from build123d import *

# Parameters (mm, degrees)
SKETCH_W        = 106.6
SKETCH_H        = 40
PAD_DEPTH       = 180
SKETCH001_W     = 102.8
SKETCH001_H     = 176.2
POCKET_DEPTH    = 38.1
SKETCH002_W     = 102.8
SKETCH002_H     = 1.9
POCKET001_DEPTH = 38.1
SKETCH003_W     = 50
SKETCH003_H     = 15
POCKET002_DEPTH = 5
SKETCH004_W     = 22
SKETCH004_H     = 20
POCKET003_DEPTH = 5
SKETCH005_W     = 75
SKETCH005_H     = 22
POCKET004_DEPTH = 5
SKETCH006_R     = 4
SKETCH006_R_2   = 4.25
POCKET005_DEPTH = 5
CHAMFER_SIZE    = 5
CHAMFER001_SIZE = 5
SKETCH007_W     = 5
SKETCH007_H     = 10
POCKET006_DEPTH = 5
SKETCH008_W     = 5
SKETCH008_H     = 10
POCKET007_DEPTH = 5
SKETCH009_W     = 19.8
SKETCH009_H     = 10
POCKET008_DEPTH = 5
SKETCH010_W     = 40
SKETCH010_H     = 5
PAD001_DEPTH    = 5
CHAMFER002_SIZE = 3.099
CHAMFER003_SIZE = 3
SKETCH011_W     = 40
SKETCH011_H     = 5
PAD002_DEPTH    = 5
CHAMFER004_SIZE = 3.099
CHAMFER005_SIZE = 3
SKETCH012_W     = 3.5
SKETCH012_H     = 22
POCKET009_DEPTH = 5
SKETCH013_W     = 3.5
SKETCH013_H     = 22
POCKET010_DEPTH = 5
SKETCH014_W     = 29
SKETCH014_H     = 50
POCKET011_DEPTH = 5
SKETCH015_W     = 102.8
SKETCH015_H     = 12
POCKET012_DEPTH = 5
SKETCH016_W     = 10
SKETCH016_H     = 12.5
POCKET013_DEPTH = 5
SKETCH017_W     = 40
SKETCH017_H     = 4
PAD003_DEPTH    = 4
CHAMFER006_SIZE = 3.099
CHAMFER007_SIZE = 1.99
SKETCH018_R     = 2.5
POCKET014_DEPTH = 5
SKETCH019_W     = 10
SKETCH019_H     = 8
POCKET015_DEPTH = 5


with BuildPart() as part:
    # Sketch → Pad (new body)
    with BuildSketch(Plane.XY):
        Rectangle(SKETCH_W, SKETCH_H)
    extrude(amount=PAD_DEPTH)

    # Sketch001 (on Face1 of Pad) → Pocket (cut)
    with BuildSketch(Plane(origin=(0, 20, 0), x_dir=(-1, 0, 0), z_dir=(0, 1, 0))):
        with Locations((0, 90)):
            Rectangle(SKETCH001_W, SKETCH001_H)
    extrude(amount=-POCKET_DEPTH, mode=Mode.SUBTRACT)

    # Sketch002 (on Face1 of Pocket) → Pocket001 (cut)
    with BuildSketch(Plane(origin=(0, 20, 0), x_dir=(-1, 0, 0), z_dir=(0, 1, 0))):
        with Locations((0, 0.95)):
            Rectangle(SKETCH002_W, SKETCH002_H)
    extrude(amount=-POCKET001_DEPTH, mode=Mode.SUBTRACT)

    # Sketch003 (on Face11 of Pocket001) → Pocket002 (cut)
    with BuildSketch(Plane.XZ.offset(20)):
        with Locations((0, 7.5)):
            Rectangle(SKETCH003_W, SKETCH003_H)
    extrude(amount=-POCKET002_DEPTH, mode=Mode.SUBTRACT)

    # Sketch004 (on Face9 of Pocket002) → Pocket003 (cut)
    with BuildSketch(Plane.YZ.offset(53.3)):
        with Locations((0, 57.78728)):
            Rectangle(SKETCH004_W, SKETCH004_H)
    extrude(amount=-POCKET003_DEPTH, mode=Mode.SUBTRACT)

    # Sketch005 (on Face10 of Pocket003) → Pocket004 (cut)
    with BuildSketch(Plane.XY.offset(180)):
        Rectangle(SKETCH005_W, SKETCH005_H)
    extrude(amount=-POCKET004_DEPTH, mode=Mode.SUBTRACT)

    # Sketch006 (on Face12 of Pocket004) → Pocket005 (cut)
    with BuildSketch(Plane.XZ.offset(20)):
        with Locations((39.85, 19.5)):
            Circle(SKETCH006_R)
        with Locations((39.85, 38.2)):
            Circle(SKETCH006_R_2)
    extrude(amount=-POCKET005_DEPTH, mode=Mode.SUBTRACT)

    # Chamfer
    chamfer_edges = [part.edges().sort_by_distance(p)[0] for p in [
        (-51.4, -18.1, 90),
        (-51.4, 0.95, 178.1),
        (0, -18.1, 178.1),
        (51.4, -18.1, 90),
        (51.4, 0.95, 178.1),
    ]]
    chamfer(chamfer_edges, length=CHAMFER_SIZE)

    # Chamfer001
    chamfer001_edges = [part.edges().sort_by_distance(p)[0] for p in [
        (53.3, -20, 90),
        (-53.3, -20, 90),
        (0, -20, 180),
        (53.3, 0, 180),
        (-53.3, 0, 180),
    ]]
    chamfer(chamfer001_edges, length=CHAMFER001_SIZE)

    # Sketch007 (on Face9 of Chamfer001) → Pocket006 (cut)
    with BuildSketch(Plane.YZ.offset(53.3)):
        with Locations((7.5, 145)):
            Rectangle(SKETCH007_W, SKETCH007_H)
        with Locations((7.5, 35)):
            Rectangle(SKETCH007_W, SKETCH007_H)
    extrude(amount=-POCKET006_DEPTH, mode=Mode.SUBTRACT)

    # Sketch008 (on Face2 of Pocket006) → Pocket007 (cut)
    with BuildSketch(Plane(origin=(-53.3, 0, 0), x_dir=(0, -1, 0), z_dir=(-1, 0, 0))):
        with Locations((-7.5, 145)):
            Rectangle(SKETCH008_W, SKETCH008_H)
        with Locations((-7.5, 35)):
            Rectangle(SKETCH008_W, SKETCH008_H)
    extrude(amount=-POCKET007_DEPTH, mode=Mode.SUBTRACT)

    # Sketch009 (on Face2 of Pocket007) → Pocket008 (cut)
    with BuildSketch(Plane(origin=(-53.3, 0, 0), x_dir=(0, -1, 0), z_dir=(-1, 0, 0))):
        with Locations((-10.1, 17.5)):
            Rectangle(SKETCH009_W, SKETCH009_H)
    extrude(amount=-POCKET008_DEPTH, mode=Mode.SUBTRACT)

    # Sketch010 (on Face4 of Pocket008) → Pad001 (join)
    with BuildSketch(Plane.YZ.offset(-51.4)):
        with Locations((0, 2.5)):
            Rectangle(SKETCH010_W, SKETCH010_H)
    extrude(amount=PAD001_DEPTH)

    # Chamfer002
    chamfer002_edges = [part.edges().sort_by_distance(p)[0] for p in [
        (-51.4, -20, 2.5),
    ]]
    chamfer(chamfer002_edges, length=CHAMFER002_SIZE)

    # Chamfer003
    chamfer003_edges = [part.edges().sort_by_distance(p)[0] for p in [
        (-46.4, 0.95, 5),
    ]]
    chamfer(chamfer003_edges, length=CHAMFER003_SIZE)

    # Sketch011 (on Face27 of Chamfer003) → Pad002 (join)
    with BuildSketch(Plane(origin=(51.4, 0, 0), x_dir=(0, -1, 0), z_dir=(-1, 0, 0))):
        with Locations((0, 2.5)):
            Rectangle(SKETCH011_W, SKETCH011_H)
    extrude(amount=PAD002_DEPTH)

    # Chamfer004
    chamfer004_edges = [part.edges().sort_by_distance(p)[0] for p in [
        (51.4, -20, 2.5),
    ]]
    chamfer(chamfer004_edges, length=CHAMFER004_SIZE)

    # Chamfer005
    chamfer005_edges = [part.edges().sort_by_distance(p)[0] for p in [
        (46.4, 0.95, 5),
    ]]
    chamfer(chamfer005_edges, length=CHAMFER005_SIZE)

    # Sketch012 (on Face15 of Chamfer005) → Pocket009 (cut)
    with BuildSketch(Plane.YZ.offset(53.3)):
        with Locations((18.25, 102)):
            Rectangle(SKETCH012_W, SKETCH012_H)
    extrude(amount=-POCKET009_DEPTH, mode=Mode.SUBTRACT)

    # Sketch013 (on Face52 of Pocket009) → Pocket010 (cut)
    with BuildSketch(Plane(origin=(-53.3, 0, 0), x_dir=(0, -1, 0), z_dir=(-1, 0, 0))):
        with Locations((-18.25, 102)):
            Rectangle(SKETCH013_W, SKETCH013_H)
    extrude(amount=-POCKET010_DEPTH, mode=Mode.SUBTRACT)

    # Sketch014 (on Face52 of Pocket010) → Pocket011 (cut)
    with BuildSketch(Plane(origin=(-53.3, 0, 0), x_dir=(0, -1, 0), z_dir=(-1, 0, 0))):
        with Locations((-5.5, 101)):
            Rectangle(SKETCH014_W, SKETCH014_H)
    extrude(amount=-POCKET011_DEPTH, mode=Mode.SUBTRACT)

    # Sketch015 (on Face6 of Pocket011) → Pocket012 (cut)
    with BuildSketch(Plane(origin=(0, 0, 0), x_dir=(1, 0, 0), z_dir=(0, 0, -1))):
        with Locations((0, -14)):
            Rectangle(SKETCH015_W, SKETCH015_H)
    extrude(amount=-POCKET012_DEPTH, mode=Mode.SUBTRACT)

    # Sketch016 (on Face37 of Pocket012) → Pocket013 (cut)
    with BuildSketch(Plane(origin=(-53.3, 0, 0), x_dir=(0, -1, 0), z_dir=(-1, 0, 0))):
        with Locations((-15, 6.25)):
            Rectangle(SKETCH016_W, SKETCH016_H)
    extrude(amount=-POCKET013_DEPTH, mode=Mode.SUBTRACT)

    # Sketch017 (on Face32 of Pocket013) → Pad003 (join)
    with BuildSketch(Plane.YZ.offset(-51.4)):
        with Locations((0, 71)):
            Rectangle(SKETCH017_W, SKETCH017_H)
        with Locations((0, 131)):
            Rectangle(SKETCH017_W, SKETCH017_H)
    extrude(amount=PAD003_DEPTH)

    # Chamfer006
    chamfer006_edges = [part.edges().sort_by_distance(p)[0] for p in [
        (-51.4, -20, 131),
        (-51.4, -20, 71),
    ]]
    chamfer(chamfer006_edges, length=CHAMFER006_SIZE)

    # Chamfer007
    chamfer007_edges = [part.edges().sort_by_distance(p)[0] for p in [
        (-47.4, 1.45, 129),
        (-47.4, 1.45, 133),
        (-47.4, 1.45, 73),
        (-47.4, 1.45, 69),
    ]]
    chamfer(chamfer007_edges, length=CHAMFER007_SIZE)

    # Sketch018 (on Face66 of Chamfer007) → Pocket014 (cut)
    with BuildSketch(Plane.XZ.offset(20)):
        with Locations((8.85, 19.5)):
            Circle(SKETCH018_R)
    extrude(amount=-POCKET014_DEPTH, mode=Mode.SUBTRACT)

    # Sketch019 (on Face8 of Pocket014) → Pocket015 (cut)
    with BuildSketch(Plane.YZ.offset(-51.4)):
        with Locations((15, 72)):
            Rectangle(SKETCH019_W, SKETCH019_H)
    extrude(amount=POCKET015_DEPTH, mode=Mode.SUBTRACT)


solid = part.part
Could you check a few things on this model? Use its own coordinates, in mm. A direction names the side the tool comes from. Give positions to 0.01 mm unless a question says otherwise; leave off trailing zeros. Order: outer loops, then holes, each group sorted by start corner. A loop starts at its lowest first (then second) coordinate and runs counter-clockwise, first axis right, second up. Notation, with made-up numbers: M -15,87.5 L 35,87.5 A26 cw 35,101.5 Z; hole C 69.25,72 d2. An arc over 180 degrees is marked long. One line per question, with ' | ' between items.
1. If I drill on line 1 (X direction, y = -13, z = 78); line 2 (Z direction, x = 39.85, y = -19.5); line 3 (X direction, y = -19, z = 19), over which ranges is the centre line in solid material (lowest first)?
Results:
line 1: -53.3 to -51.4, 51.4 to 53.3 | line 2: 0 to 15.5, 23.5 to 33.95, 42.45 to 175.5 | line 3: -49.3 to 6.4, 11.3 to 35.88, 43.82 to 49.3
2. I want a section at B-B (z = 19.5). List the corners of the cut face in (x, y) for me.
Results:
outline: M -53.3,-15 L -48.3,-20 L 6.35,-20 L 6.35,-18.1 L -46.4,-18.1 L -51.4,-13.1 L -51.4,0.2 L -53.3,0.2 Z; M 11.35,-20 L 35.85,-20 L 35.85,-18.1 L 11.35,-18.1 Z; M 43.85,-20 L 48.3,-20 L 53.3,-15 L 53.3,20 L 51.4,20 L 51.4,-13.1 L 46.4,-18.1 L 43.85,-18.1 Z
3. I want a section at D-D (y = -5). Give the number of separate pieces and of enclosed holes in the cut face, and give its area (3 significant figures).
Results:
separate pieces: 4 | enclosed holes: 0 | area: 669 mm²
4. For faces 1 (the face through (48.9, -15.6, 86.4)), 2 (the face through (-47, -7, 0)), 3 (the face through (49, 8, 2)), which set-ups out of +Z, -Z, +X, -X, +Y, -Y let a thin tool reach every point of the face, with its end or its side?
Results:
face 1: +Y | face 2: -Z, +X, -X, +Y, -Y | face 3: -Z, +Y
5. We'd pull the mould along Z, two halves only. Please class faces 4 (the face through (-49.8, -16.6, 176.9)), 5 (the face through (1, 15, 178.1)), 6 (the face through (48.3, -14.7, 174.6)): +Z half, -Z half, draft (parallel to the pull), parting line (faces both ways), or undercut.
Results:
face 4: +Z half | face 5: -Z half | face 6: undercut
6. I want a section at A-A (x = 8.85). List the corners of the cut face in (y, z) for me.
Results:
outline: M -20,15 L -18.1,15 L -18.1,17 L -20,17 Z; M -20,22 L -18.1,22 L -18.1,173.1 L -13.1,178.1 L -11,178.1 L -11,180 L -15,180 L -20,175 Z; M 11,178.1 L 20,178.1 L 20,180 L 11,180 Z
7. I'm going to push flat-ended pins straight in: pin 1 (12 mm diameter, centred on x = 37.5, y = -6, fed in from -Z); pin 2 (6 mm diameter, centred on x = 18.5, y = -11.5, fed in from -Z); pin 3 (8 mm diameter, centred on x = 13, z = 93, fed in from +Y); pin 4 (1.5 mm diameter, centred on x = -52, y = 8, fed in from -Z). Where does each tip first touch, or does it pass through?
Results:
pin 1: z = 178.1 | pin 2: z = 176.7 | pin 3: y = -18.1 | pin 4: z = 0
8. I want a section at C-C (z = 53). List the corners of the cut face in (x, y) for me, and give its area (3 significant figures).
Results:
outline: M -53.3,-15 L -48.3,-20 L 48.3,-20 L 53.3,-15 L 53.3,-11 L 51.4,-11 L 51.4,-13.1 L 46.4,-18.1 L -46.4,-18.1 L -51.4,-13.1 L -51.4,20 L -53.3,20 Z; M 51.4,11 L 53.3,11 L 53.3,20 L 51.4,20 Z | area: 306 mm²
